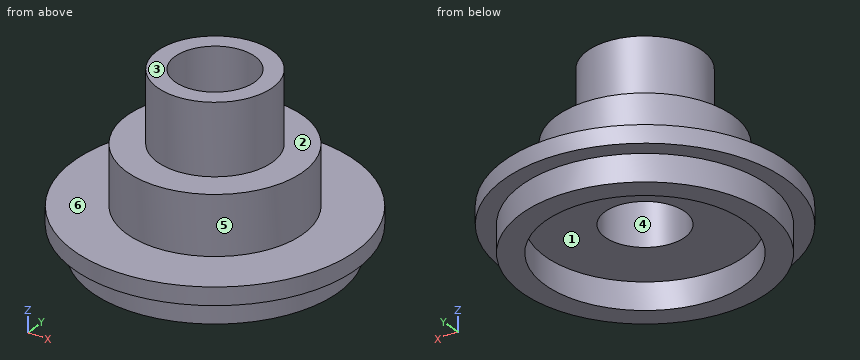
```python
from build123d import *

# Parameters (mm, degrees)
F2_R     = 4.9
F3_DEPTH = 6
F4_R     = 3.4
F5_DEPTH = 14.801


with BuildPart() as f1:
    # F0 (on Right) → F1 (revolve)
    with BuildSketch(Plane.YZ):
        Polygon((0, 6.5), (0, 0), (8.5, 0), (8.5, -2.3), (10.5, -2.3), (10.5, 0), (12, 0), (12, 1.5), (7.5, 1.5), (7.5, 6.5), align=None)
    revolve(axis=Axis((0, 0, 3.25), (0, 0, -1)))

    # F2 (on face) → F3 (join)
    with BuildSketch(Plane.XY.offset(6.5)):
        Circle(F2_R)
    extrude(amount=F3_DEPTH)

    # F4 (on face) → F5 (cut, through all)
    with BuildSketch(Plane.XY.offset(12.5)):
        Circle(F4_R)
    extrude(amount=-F5_DEPTH, mode=Mode.SUBTRACT)


solid = f1.part
```
Read the model definition and answer for the solid it produces. Units are mm, in the model's axes. Face numbers are marked on the shaded views. A direction names the side the tool comes from. Give positions to 0.01 mm unless a question says otherwise; leave off trailing zeros. Write each loop counter-clockwise with the first axis right and the second up, starting at its lowest first coordinate (ties: lowest second). Pieces come first, ordered by that corner, then holes. Notation, with made-up numbers: (47.5, 57) - (97.5, 57) arc R30 cw to (97.5, 86) - close; hole circle Ø2 at (-40, 84). An arc over 180 degrees is marked (long way). Write item = value, one per line. Start each with the question number.
Item 1: The mould has two halves that part along X. Classify the marked faces 4, 5 and 6: +X half, -X half, draft (parallel to the pull), parting line (faces both ways), or undercut.
Item 2: A tool of negligible diameter and unlimited length cuts with its end or side. For the marked faces 1, 2 and 3, from which of +Z, -Z, +X, -X, +Y, -Y can it reach the whole face along a straight path? Write none if from no direction.
Item 3: Find section C-C (z = 3.5). Give the vertices of the cut face in (x, y), then the cut area to 3 significant figures.
Item 4: Find the intervals of material crossed by probe 1 along X at (y, z) = (0, -1.35); probe 2 along Z at (x, y) = (-1, -7.5); probe 3 along Z at (x, y) = (9.75, 3.5), in increasing order. Write a range as [from, to].
Item 5: Find section A-A (y = 0). Give the vertices of the cut face in (x, z).
Item 6: Find section D-D (x = 6.75). Give the vertices of the cut face in (y, z).
Item 7: Each of these flat-tipped pins is pushed along its axis until it touches: P1, Ø2, axis at x = 6, z = 10, coming from the +Y side; P2, Ø3, axis at x = 7, z = 0, coming from the +Y side; P3, Ø1.5, axis at x = -3.5, z = 5.5, coming from the +Y side; P4, Ø6, axis at y = -5.5, z = 3, coming from the -X side. Where does it stop, or does it pass through?
Response:
q1.face_4 = undercut
q1.face_5 = parting line
q1.face_6 = draft
q2.face_1 = -Z
q2.face_2 = +Z
q2.face_3 = +Z, +X, -X, +Y, -Y
q3.outline = circle Ø15 at (0, 0); hole circle Ø6.8 at (0, 0)
q3.area = 140 mm²
q4.probe_1 = [-10.5, -8.5], [8.5, 10.5]
q4.probe_2 = [0, 1.5]
q4.probe_3 = [-2.3, 1.5]
q5.outline = (-12, 0) - (-10.5, 0) - (-10.5, -2.3) - (-8.5, -2.3) - (-8.5, 0) - (-3.4, 0) - (-3.4, 12.5) - (-4.9, 12.5) - (-4.9, 6.5) - (-7.5, 6.5) - (-7.5, 1.5) - (-12, 1.5) - close; (3.4, 0) - (8.5, 0) - (8.5, -2.3) - (10.5, -2.3) - (10.5, 0) - (12, 0) - (12, 1.5) - (7.5, 1.5) - (7.5, 6.5) - (4.9, 6.5) - (4.9, 12.5) - (3.4, 12.5) - close
q6.outline = (-9.92, 0) - (-8.04, 0) - (-8.04, -2.3) - (-5.17, -2.3) - (-5.17, 0) - (5.17, 0) - (5.17, -2.3) - (8.04, -2.3) - (8.04, 0) - (9.92, 0) - (9.92, 1.5) - (3.27, 1.5) - (3.27, 6.5) - (-3.27, 6.5) - (-3.27, 1.5) - (-9.92, 1.5) - close
q7.P1 = through
q7.P2 = 10.67
q7.P3 = 6.98
q7.P4 = -11.64
